Verification items for the finished model (mm, model axes). Face numbers are marked on the shaded views. A direction names the side the tool comes from. Round coordinates to 2 decimals unless told otherwise and drop trailing zeros. Order: outer loops, then holes, each group sorted by start corner. A loop starts at its lowest first (then second) coordinate and runs counter-clockwise, first axis right, second up. Notation, with made-up numbers: (43, 20.25) -> (92, 20.25) arc R10 cw to (92, 27.25) -> close; hole circle Ø1 at (12.5, 71). An arc over 180 degrees is marked (long way). Put each result on its own line as item: value.
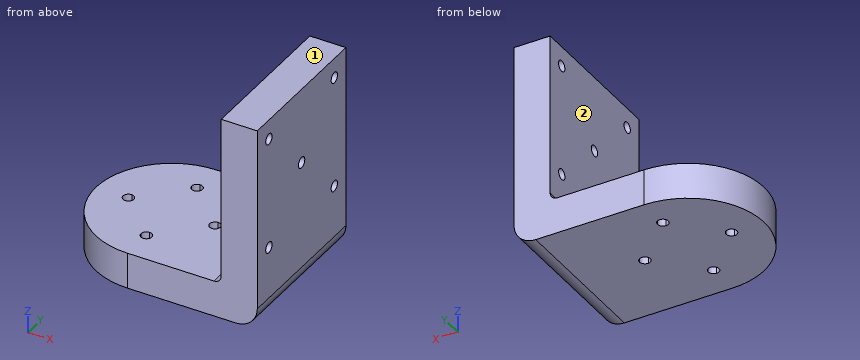
```python
from build123d import *

# Parameters (mm, degrees)
SKETCH_1_W      = 5
SKETCH_1_H      = 42
EXTRUDE_1_DEPTH = 10
SKETCH_2_W      = 57
SKETCH_2_H      = 42
SKETCH_2_R      = 1.5
EXTRUDE_2_DEPTH = 10
FILLET_1_R      = 2
FILLET_2_R      = 6


with BuildPart() as part:
    # 草图1 → 凸台-拉伸1 (new body)
    with BuildSketch(Plane.XY):
        with BuildLine():
            Line((0, 13.5), (0, 21))
            ThreePointArc((0, 21), (-21, 0), (0, -21))
            Line((0, -21), (0, -13.5))
            ThreePointArc((0, -13.5), (-1.09330348, -13.026979795), (-1.497067446, -11.90625))
            ThreePointArc((-1.497067446, -11.90625), (-8.485281374, -8.485281374), (-11.90625, -1.497067446))
            ThreePointArc((-11.90625, -1.497067446), (-13.5, 0), (-11.90625, 1.497067446))
            ThreePointArc((-11.90625, 1.497067446), (-8.485281374, 8.485281374), (-1.497067446, 11.90625))
            ThreePointArc((-1.497067446, 11.90625), (-1.09330348, 13.026979795), (0, 13.5))
        make_face()
        with BuildLine():
            ThreePointArc((21, 0), (14.849242405, 14.849242405), (0, 21))
            Line((0, 21), (0, 13.5))
            ThreePointArc((0, 13.5), (1.060660172, 13.060660172), (1.5, 12))
            ThreePointArc((1.5, 12), (1.499266682, 11.953102073), (1.497067446, 11.90625))
            ThreePointArc((1.497067446, 11.90625), (8.485281374, 8.485281374), (11.90625, 1.497067446))
            ThreePointArc((11.90625, 1.497067446), (13.026979795, 1.09330348), (13.5, 0))
            ThreePointArc((13.5, 0), (13.026979795, -1.09330348), (11.90625, -1.497067446))
            ThreePointArc((11.90625, -1.497067446), (8.485281374, -8.485281374), (1.497067446, -11.90625))
            ThreePointArc((1.497067446, -11.90625), (1.499266682, -11.953102073), (1.5, -12))
            ThreePointArc((1.5, -12), (1.060660172, -13.060660172), (0, -13.5))
            Line((0, -13.5), (0, -21))
            ThreePointArc((0, -21), (14.849242405, -14.849242405), (21, 0))
        make_face()
        with BuildLine():
            ThreePointArc((0, 10.5), (-1.026979795, 10.90669652), (-1.497067446, 11.90625))
            ThreePointArc((-1.497067446, 11.90625), (-8.485281374, 8.485281374), (-11.90625, 1.497067446))
            ThreePointArc((-11.90625, 1.497067446), (-10.90669652, 1.026979795), (-10.5, 0))
            ThreePointArc((-10.5, 0), (-10.90669652, -1.026979795), (-11.90625, -1.497067446))
            ThreePointArc((-11.90625, -1.497067446), (-8.485281374, -8.485281374), (-1.497067446, -11.90625))
            ThreePointArc((-1.497067446, -11.90625), (-1.026979795, -10.90669652), (0, -10.5))
            Line((0, -10.5), (0, 10.5))
        make_face()
        with BuildLine():
            ThreePointArc((1.497067446, 11.90625), (1.026979795, 10.90669652), (0, 10.5))
            Line((0, 10.5), (0, -10.5))
            ThreePointArc((0, -10.5), (1.026979795, -10.90669652), (1.497067446, -11.90625))
            ThreePointArc((1.497067446, -11.90625), (8.485281374, -8.485281374), (11.90625, -1.497067446))
            ThreePointArc((11.90625, -1.497067446), (10.5, 0), (11.90625, 1.497067446))
            ThreePointArc((11.90625, 1.497067446), (8.485281374, 8.485281374), (1.497067446, 11.90625))
        make_face()
        with BuildLine():
            Line((21, 21), (0, 21))
            ThreePointArc((0, 21), (14.849242405, 14.849242405), (21, 0))
            Line((21, 0), (21, 21))
        make_face()
        with Locations((23.5, 0)):
            Rectangle(SKETCH_1_W, SKETCH_1_H)
        Polygon((26, 21), (21, 21), (21, 0), (21, -21), (26, -21), align=None)
        with BuildLine():
            Line((21, -21), (21, 0))
            ThreePointArc((21, 0), (14.849242405, -14.849242405), (0, -21))
            Line((0, -21), (21, -21))
        make_face()
    extrude(amount=EXTRUDE_1_DEPTH)

    # 草图2 → 凸台-拉伸2 (add)
    with BuildSketch(Plane(origin=(26, 0, 0), x_dir=(0, 0, -1), z_dir=(1, 0, 0))):
        with Locations((-28.5, 0)):
            Rectangle(SKETCH_2_W, SKETCH_2_H)
        with Locations((-51.5, 15.5)):
            Circle(SKETCH_2_R, mode=Mode.SUBTRACT)
        with Locations((-36, 0)):
            Circle(SKETCH_2_R, mode=Mode.SUBTRACT)
        with Locations((-51.5, -15.5)):
            Circle(SKETCH_2_R, mode=Mode.SUBTRACT)
        with Locations((-20.5, -15.5)):
            Circle(SKETCH_2_R, mode=Mode.SUBTRACT)
        with Locations((-20.5, 15.5)):
            Circle(SKETCH_2_R, mode=Mode.SUBTRACT)
    extrude(amount=EXTRUDE_2_DEPTH)

    # 圆角1
    fillet_1_edges = [part.edges().sort_by_distance(p)[0] for p in [
        (26, 0, 10),
    ]]
    fillet(fillet_1_edges, radius=FILLET_1_R)

    # 圆角2
    fillet_2_edges = [part.edges().sort_by_distance(p)[0] for p in [
        (36, 0, 0),
    ]]
    fillet(fillet_2_edges, radius=FILLET_2_R)


solid = part.part
```
Item 1: Depth check by flat-ended pin: pin 1 Ø4 at (y, z) = (15.5, 51.5) entering from -X; pin 2 Ø8 at (x, z) = (-13, 10) entering from -Y; pin 3 Ø1 at (x, y) = (-8, 8.5) entering from +Z. Enter the tip coordinate at first touch or a pass-through.
Geometry check:
pin 1: x = 26
pin 2: y = -18.97
pin 3: z = 10
Item 2: Sectioned sample at D-D, the plane z = 7. Record the boundary of the cut face in (x, y).
Geometry check:
outline: (0, -21) -> (36, -21) -> (36, 21) -> (0, 21) arc R21 ccw to start; hole circle Ø3 at (-12, 0); hole circle Ø3 at (0, -12); hole circle Ø3 at (0, 12); hole circle Ø3 at (12, 0)
Item 3: Sectioned sample at B-B, the plane y = 15.5. Record the boundary of the cut face in (x, z).
Geometry check:
outline: (-14.17, 0) -> (30, 0) arc R6 ccw to (36, 6) -> (36, 19) -> (26, 19) -> (26, 12) arc R2 cw to (24, 10) -> (-14.17, 10) -> close; (26, 22) -> (36, 22) -> (36, 50) -> (26, 50) -> close; (26, 53) -> (36, 53) -> (36, 57) -> (26, 57) -> close
Item 4: Sectioned sample at C-C, the plane x = 32. Record the boundary of the cut face in (y, z), then the cut area to 3 significant figures.
Geometry check:
outline: (-21, 0.34) -> (21, 0.34) -> (21, 57) -> (-21, 57) -> close; hole circle Ø3 at (-15.5, 20.5); hole circle Ø3 at (-15.5, 51.5); hole circle Ø3 at (0, 36); hole circle Ø3 at (15.5, 20.5); hole circle Ø3 at (15.5, 51.5)
area: 2,340 mm2
Item 5: Tool access check on the marked faces 1 and 2. Record the directions out of +Z, -Z, +X, -X, +Y, -Y that give a thin tool (end or side, any length) a straight path to the whole face; none if there is none.
Geometry check:
face 1: +Z, +X, -X, +Y, -Y
face 2: +Z, -X, +Y, -Y
Item 6: Material ranges on line 1 along Y through (x, z) = (28.25, 20.5); line 2 along Y through (x, z) = (33, 20); line 3 along X through (y, z) = (-1, 24), recorded low to high.
Geometry check:
line 1: -21 to -17, -14 to 14, 17 to 21
line 2: -21 to -16.91, -14.09 to 14.09, 16.91 to 21
line 3: 26 to 36
Item 7: Sectioned sample at A-A, the plane z = 20.5. Record the boundary of the cut face in (x, y).
Geometry check:
outline: (26, -21) -> (36, -21) -> (36, -17) -> (26, -17) -> close; (26, -14) -> (36, -14) -> (36, 14) -> (26, 14) -> close; (26, 17) -> (36, 17) -> (36, 21) -> (26, 21) -> close
